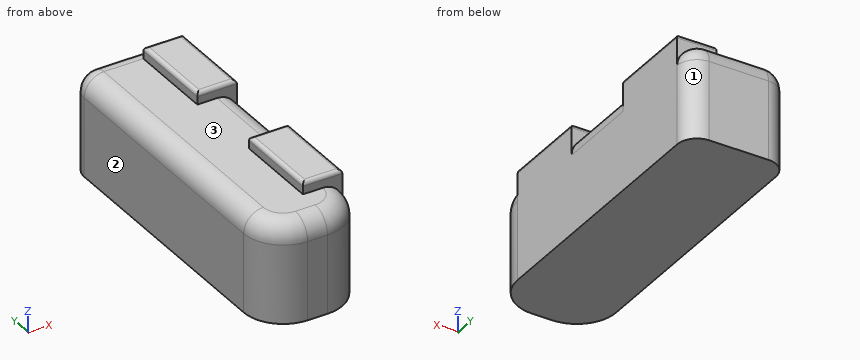
from build123d import *

# Parameters (mm, degrees)
F1_DEPTH = 25
F2_W     = 10
F2_H     = 22
F3_DEPTH = 3
F4_R     = 4.99999
F5_R     = 1


# Not quite as in the source:
# - a fillet or chamfer is up to 0.001 mm smaller than in the source, because OpenCascade refuses the exact size


with BuildPart() as f1:
    # F0 (on Top) → F1 (new body)
    with BuildSketch(Plane.XY):
        with BuildLine():
            Line((0, 54.0433624494), (0, 53.3714158042))
            Line((0, 53.3714158042), (25, 53.3714158042))
            Line((25, 53.3714158042), (25, 54.0433624494))
            ThreePointArc((25, 54.0433624494), (23.5355339059, 57.5788963554), (20, 59.0433624494))
            Line((20, 59.0433624494), (5, 59.0433624494))
            ThreePointArc((5, 59.0433624494), (1.4644660941, 57.5788963554), (0, 54.0433624494))
        make_face()
        with BuildLine():
            Line((25, 53.3714158042), (0, 53.3714158042))
            Line((0, 53.3714158042), (0, -10.9566375506))
            ThreePointArc((0, -10.9566375506), (2.9289321881, -18.0277053624), (10, -20.9566375506))
            Line((10, -20.9566375506), (15, -20.9566375506))
            ThreePointArc((15, -20.9566375506), (22.0710678119, -18.0277053624), (25, -10.9566375506))
            Line((25, -10.9566375506), (25, 53.3714158042))
        make_face()
    extrude(amount=F1_DEPTH)

    # F2 (on face) → F3 (join)
    with BuildSketch(Plane.XY.offset(25)):
        with Locations((20, 0.0433624494)):
            Rectangle(F2_W, F2_H)
        with Locations((20, 43.0433624494)):
            Rectangle(F2_W, F2_H)
    extrude(amount=F3_DEPTH)

    # F4 (radius 5 in the source; OpenCascade refuses exactly that, so slightly less here)
    f4_edges = [f1.edges().sort_by_distance(p)[0] for p in [
        (25, 21.543362, 25),
        (0, 21.543362, 25),
    ]]
    fillet(f4_edges, radius=F4_R)

    # F5
    f5_edges = [f1.edges().sort_by_distance(p)[0] for p in [
        (15, 0.043362, 28),
        (20, -10.956638, 28),
        (25, 0.043362, 28),
        (20, 11.043362, 28),
        (25, 43.043362, 28),
        (20, 54.043362, 28),
        (15, 43.043362, 28),
        (20, 32.043362, 28),
    ]]
    fillet(f5_edges, radius=F5_R)


solid = f1.part
CAD build for the part. Positions are in the model's coordinates, mm. Face numbers are marked on the shaded views. Round coordinates to 2 decimals unless told otherwise and drop trailing zeros. Write each loop counter-clockwise with the first axis right and the second up, starting at its lowest first coordinate (ties: lowest second). Pieces come first, ordered by that corner, then holes. Notation, with made-up numbers: M -37,1.5 L 13,1.5 A17 cw 13,12.5 Z; hole C 32,85.5 d3. An arc over 180 degrees is marked long. Use a Markdown table: item, result. Add a question column.
1. Flat gauge pins, fed straight in: P1, Ø3.5, axis at x = 20.5, z = 24.5, coming from the -Y side; P2, Ø2, axis at y = 47.5, z = 25.5, coming from the -X side; P3, Ø2, axis at x = 18.5, z = 24.5, coming from the -Y side. Where does each tip first touch, or does it go through?
2. Slice it at C-C on z = 8. Give the cut face in (x, y), then the cut area to 3 significant figures.
3. Drill centre lines: probe 1 along Z at (x, y) = (7.5, 36); probe 2 along Y at (x, z) = (12.25, 20.25); probe 3 along Y at (x, z) = (3.5, 2.5). Where is each one in solid material? Low to high.
4. Pull direction Y, two halves, no side cores. Call the marked faces 1, 2 and 3: released by +Y, released by -Y, zero draft, split by the parting line, or undercut.
5. Slice it at A-A on y = 47. Give the cut face in (x, z).
6. Slice it at B-B on x = 14.25. Give the cut face in (y, z), then the cut area to 3 significant figures.
7. Slice it at D-D on y = 19. Give the cut face in (x, z), then the cut area to 3 significant figures.
Reply:
| question | item | result |
|---|---|---|
| 1 | P1 | stops at y = -18.7 |
| 1 | P2 | stops at x = 2.82 |
| 1 | P3 | stops at y = -18.86 |
| 2 | outline | M 0,-10.96 A10 ccw 10,-20.96 L 15,-20.96 A10 ccw 25,-10.96 L 25,54.04 A5 ccw 20,59.04 L 5,59.04 A5 ccw 0,54.04 Z |
| 2 | area | 1,950 mm^2 |
| 3 | probe 1 | z = 0 to 25 |
| 3 | probe 2 | y = -20.95 to 59.04 |
| 3 | probe 3 | y = -18.56 to 58.81 |
| 4 | face 1 | released by +Y |
| 4 | face 2 | zero draft |
| 4 | face 3 | undercut |
| 5 | outline | M 0,0 L 25,0 L 25,27 A1 ccw 24,28 L 16,28 A1 ccw 15,27 L 15,25 L 5,25 A5 ccw 0,20 Z |
| 6 | outline | M -20.96,0 L 59.04,0 L 59.04,20 A5 ccw 54.04,25 L -15.96,25 A5 ccw -20.96,20 Z |
| 6 | area | 1,990 mm^2 |
| 7 | outline | M 0,0 L 25,0 L 25,20 A5 ccw 20,25 L 5,25 A5 ccw 0,20 Z |
| 7 | area | 614 mm^2 |
